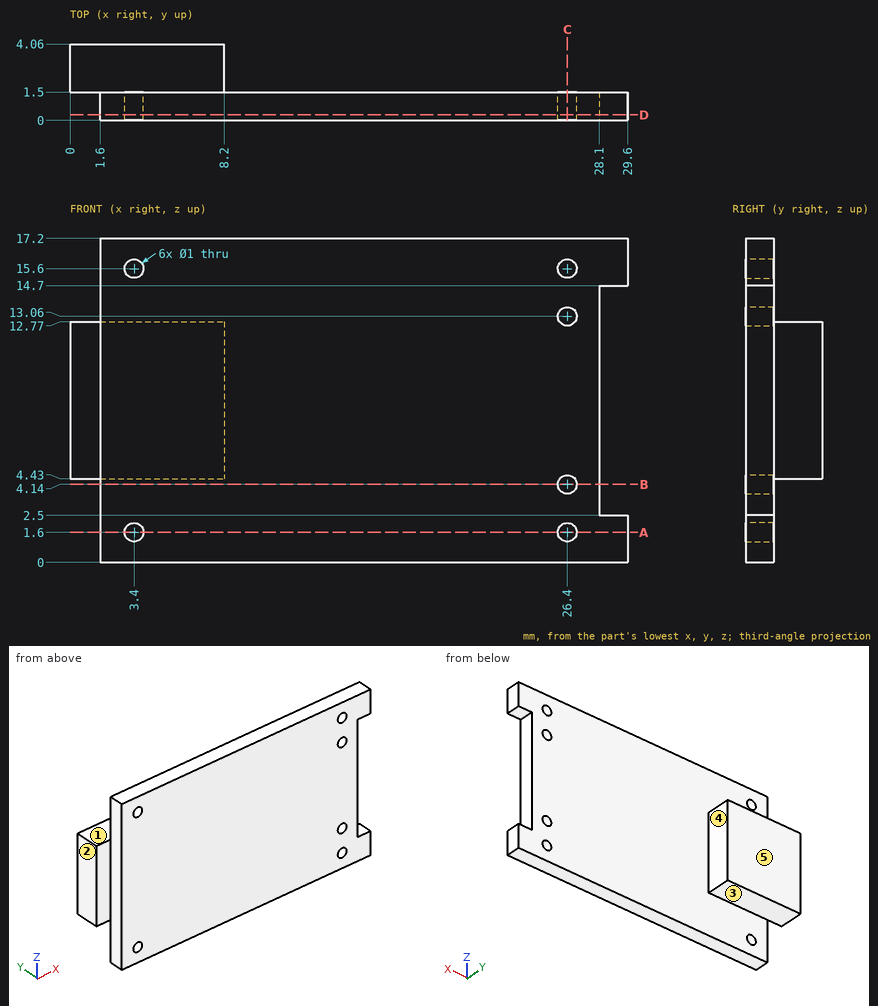
Answer from the drawing. Dimensions are ordinates in mm from the lowest x, y and z of the part. A direction names the side the tool comes from. Give positions to 0.01 mm unless a question says otherwise; leave off trailing zeros. Write each loop counter-clockwise with the first axis right and the second up, starting at its lowest first coordinate (ties: lowest second). Pieces come first, ordered by that corner, then holes.
1) Section B-B (z = 4.14) is taken. Write down the section's boundary in (x, y).
2) Section D-D (y = 0.3) is taken. Write down the section's boundary in (x, z), and give its area (3 significant figures).
3) Section A-A (z = 1.6) is taken. Write down the section's boundary in (x, y), and give its area (3 significant figures).
4) Given P1, Ø1, axis at x = 12, y = 0.5, coming from the -Z side; P2, Ø0.8, axis at y = 1, z = 10, coming from the -X side; P3, Ø2, axis at y = 1.5, z = 7, coming from the +X side; P4, Ø0.8, axis at x = 3, y = 2.5, coming from the -Z side, each flat-ended and moving along its own axis, determine where each tip first touches the part or whether it passes through.
5) Find the intervals of material crossed by L1, parallel to X at y = 0.4, z = 15.6; L2, parallel to X at y = 0.55, z = 4.14; L3, parallel to Y at x = 18.5, z = 5.75, in increasing order.
6) Section C-C (x = 26.4) is taken. Write down the section's boundary in (y, z).
7) A tool of negligible diameter and unlimited length cuts with its end or side. For the marked faces 1, 2, 3, 4 and 5, from which of +Z, -Z, +X, -X, +Y, -Y can it reach the whole face along a straight path? Write none if from no direction.
Response:
1. outline: (1.6, 0) - (25.9, 0) - (25.9, 1.5) - (1.6, 1.5) - close; (26.9, 0) - (28.1, 0) - (28.1, 1.5) - (26.9, 1.5) - close
2. outline: (1.6, 0) - (29.6, 0) - (29.6, 2.5) - (28.1, 2.5) - (28.1, 14.7) - (29.6, 14.7) - (29.6, 17.2) - (1.6, 17.2) - close; hole circle Ø1 at (3.4, 1.6); hole circle Ø1 at (3.4, 15.6); hole circle Ø1 at (26.4, 1.6); hole circle Ø1 at (26.4, 4.14); hole circle Ø1 at (26.4, 13.06); hole circle Ø1 at (26.4, 15.6)
2. area: 459 mm2
3. outline: (1.6, 0) - (2.9, 0) - (2.9, 1.5) - (1.6, 1.5) - close; (3.9, 0) - (25.9, 0) - (25.9, 1.5) - (3.9, 1.5) - close; (26.9, 0) - (29.6, 0) - (29.6, 1.5) - (26.9, 1.5) - close
3. area: 39.0 mm2
4. P1: stops at z = 0
4. P2: stops at x = 1.6
4. P3: stops at x = 28.1
4. P4: stops at z = 4.43
5. L1: x = 1.6 to 2.9, 3.9 to 25.9, 26.9 to 29.6
5. L2: x = 1.6 to 25.9, 26.9 to 28.1
5. L3: y = 0 to 1.5
6. outline: (0, 0) - (1.5, 0) - (1.5, 1.1) - (0, 1.1) - close; (0, 2.1) - (1.5, 2.1) - (1.5, 3.64) - (0, 3.64) - close; (0, 4.64) - (1.5, 4.64) - (1.5, 12.56) - (0, 12.56) - close; (0, 13.56) - (1.5, 13.56) - (1.5, 15.1) - (0, 15.1) - close; (0, 16.1) - (1.5, 16.1) - (1.5, 17.2) - (0, 17.2) - close
7. face 1: +Z, +X, -X, +Y
7. face 2: +Z, -Z, -X, +Y, -Y
7. face 3: -Z, +X, -X, +Y
7. face 4: +Z, -Z, +X, +Y
7. face 5: +Z, -Z, +X, -X, +Y
